For this review, take the finished solid that the model builds, in its own axes (mm). A direction names the side the tool comes from. Coordinates: 2 decimals unless noted, no trailing zeros. Loops run counter-clockwise (first coordinate to the right, second up) from the corner with the lowest first, then second, coordinate; pieces in that order, holes last. Notation, with made-up numbers: (71.5, 19.25) -> (119.5, 19.25) arc R29 cw to (119.5, 46.25) -> close; hole circle Ø8 at (23, 22.5). An arc over 180 degrees is marked (long way). Use a Markdown table: item, result.
from build123d import *

# Parameters (mm, degrees)
F0_R     = 44.45
F1_DEPTH = 9.525
F2_R     = 2.0828
F3_DEPTH = 25.4
F4_R     = 3.6322
F5_DEPTH = 4.1656
F6_R     = 2.38125
F7_R     = 12.7


with BuildPart() as f1:
    # F0 (on Top) → F1 (new body)
    with BuildSketch(Plane.XY):
        with BuildLine():
            Line((-25.4, 90.4875), (-25.4, 43.994091))
            ThreePointArc((-25.4, 43.994091), (0, -50.8), (25.4, 43.994091))
            Line((25.4, 43.994091), (25.4, 90.4875))
            Line((25.4, 90.4875), (-25.4, 90.4875))
        make_face()
        Circle(F0_R, mode=Mode.SUBTRACT)
    extrude(amount=F1_DEPTH)

    # F2 (on face) → F3 (cut)
    with BuildSketch(Plane.XY.offset(9.525)):
        with Locations((-20.6375, 84.1375)):
            Circle(F2_R)
        with Locations((20.6375, 84.1375)):
            Circle(F2_R)
        with Locations((20.6375, 53.9623)):
            Circle(F2_R)
        with Locations((-20.6375, 53.9623)):
            Circle(F2_R)
        Polygon((-17.42166, 69.0499), (-8.71083, 53.9623), (8.71083, 53.9623), (17.42166, 69.0499), (8.71083, 84.1375), (-8.71083, 84.1375), align=None)
    extrude(amount=-F3_DEPTH, mode=Mode.SUBTRACT)

    # F4 (on face) → F5 (cut)
    with BuildSketch(Plane.XY.offset(9.525)):
        with Locations((-20.6375, 84.1375)):
            Circle(F4_R)
        with Locations((20.6375, 84.1375)):
            Circle(F4_R)
        with Locations((20.6375, 53.9623)):
            Circle(F4_R)
        with Locations((-20.6375, 53.9623)):
            Circle(F4_R)
    extrude(amount=-F5_DEPTH, mode=Mode.SUBTRACT)

    # F6
    f6_edges = [f1.edges().sort_by_distance(p)[0] for p in [
        (-25.4, 90.4875, 4.7625),
        (25.4, 90.4875, 4.7625),
    ]]
    fillet(f6_edges, radius=F6_R)

    # F7
    f7_edges = [f1.edges().sort_by_distance(p)[0] for p in [
        (-25.4, 43.994091, 4.7625),
        (25.4, 43.994091, 4.7625),
    ]]
    fillet(f7_edges, radius=F7_R)


solid = f1.part
(1) Mouldability with a two-part tool opening along X and no side actions: class faces 6 (the face through (19.85, 50.416, 7.471)), 7 (the face through (-25.4, 70, 5)), 8 (the face through (-18.961, 80.915, 7.471)), 9 (the face through (0, 90.488, 5)) as pulls with the +X half, pulls with the -X half, needs draft (parallel to the pull), parting line crosses it, or undercut.
Found:
| item | result |
|---|---|
| face 6 | undercut |
| face 7 | pulls with the -X half |
| face 8 | undercut |
| face 9 | needs draft |
(2) Take a section at C-C on z = 7.25. Write out the cut boundary in (x, y).
Found:
| item | result |
|---|---|
| outline | (-30.48, 40.64) arc R50.8 ccw (long way) to (30.48, 40.64) arc R12.7 cw to (25.4, 50.8) -> (25.4, 88.11) arc R2.38 ccw to (23.02, 90.49) -> (-23.02, 90.49) arc R2.38 ccw to (-25.4, 88.11) -> (-25.4, 50.8) arc R12.7 cw to start; hole circle Ø88.9 at (0, 0); hole circle Ø7.26 at (-20.64, 53.96); hole circle Ø7.26 at (-20.64, 84.14); hole (-17.42, 69.05) -> (-8.71, 53.96) -> (8.71, 53.96) -> (17.42, 69.05) -> (8.71, 84.14) -> (-8.71, 84.14) -> close; hole circle Ø7.26 at (20.64, 53.96); hole circle Ø7.26 at (20.64, 84.14) |
(3) For pin 1 Ø6.5 at (x, y) = (-20.64, 84.14) entering from -Z; pin 2 Ø4 at (x, z) = (-0.5, 7) entering from -Y; pin 3 Ø2 at (y, z) = (25, 3.5) entering from -X; pin 4 Ø2.5 at (x, y) = (-20.64, 84.14) entering from -Z, all flat-tipped, find the tip position at first contact; note any pin that passes through.
Found:
| item | result |
|---|---|
| pin 1 | stops at z = 0 |
| pin 2 | stops at y = -50.8 |
| pin 3 | stops at x = -44.77 |
| pin 4 | passes through |
(4) For line 1 along Y through (x, z) = (-1.5, 2.75); line 2 along Y through (x, z) = (-8, 9.25); line 3 along X through (y, z) = (16, 5.75), list the stretches that pass through material, from the lowest coordinate up.
Found:
| item | result |
|---|---|
| line 1 | y = -50.78 to -44.42, 44.42 to 53.96, 84.14 to 90.49 |
| line 2 | y = -50.17 to -43.72, 43.72 to 53.96, 84.14 to 90.49 |
| line 3 | x = -48.21 to -41.47, 41.47 to 48.21 |
(5) For faces 1 (the face through (-4, 46, 0)), 2 (the face through (-19, 52, 5.359)), 3 (the face through (0, 84.138, 5)), 4 (the face through (25.4, 69, 5)), 5 (the face through (-4, 46, 9.525)), list the 3-axis set-ups (+Z, -Z, +X, -X, +Y, -Y) from which the entire face can be reached by the end or side of a thin tool; tool diameter is ignored.
Found:
| item | result |
|---|---|
| face 1 | -Z, +X, -X, +Y, -Y |
| face 2 | +Z |
| face 3 | +Z, -Z |
| face 4 | +Z, -Z, +X, +Y |
| face 5 | +Z, +X, -X, +Y, -Y |
(6) Take a section at B-B on y = 0. Write out the cut boundary in (x, z) (3 decimals), plus the area to 3 significant figures.
Found:
| item | result |
|---|---|
| outline | (-50.8, 0) -> (-44.45, 0) -> (-44.45, 9.525) -> (-50.8, 9.525) -> close; (44.45, 0) -> (50.8, 0) -> (50.8, 9.525) -> (44.45, 9.525) -> close |
| area | 121 mm^2 |
(7) Take a section at A-A on x = 0. State how many separate pieces and enclosed holes the cut face has, plus the area to 3 significant figures.
Found:
| item | result |
|---|---|
| separate pieces | 3 |
| enclosed holes | 0 |
| area | 212 mm^2 |
(8) Take a section at D-D on y = 26. Write out the cut boundary in (x, z) (3 decimals), plus the area to 3 significant figures.
Found:
| item | result |
|---|---|
| outline | (-43.642, 0) -> (-36.053, 0) -> (-36.053, 9.525) -> (-43.642, 9.525) -> close; (36.053, 0) -> (43.642, 0) -> (43.642, 9.525) -> (36.053, 9.525) -> close |
| area | 145 mm^2 |
